Source: CAD feature listing. Evaluate the final solid. Frame: model axes, mm. A direction names the side the tool comes from. Round coordinates to 2 decimals unless told otherwise and drop trailing zeros. Order: outer loops, then holes, each group sorted by start corner. A loop starts at its lowest first (then second) coordinate and runs counter-clockwise, first axis right, second up.
Autodesk Inventor part; units mm, degrees
ref_plane "YZ Plane" through (0, 0, 0) normal (1, 0, 0) x (0, 1, 0)
ref_plane "XZ Plane" through (0, 0, 0) normal (0, 1, 0) x (-1, 0, 0)
ref_plane "XY Plane" through (0, 0, 0) normal (0, 0, 1) x (1, 0, 0)
ref_plane "Arbeitsebene1" through (-0.5, 0, -8) normal (0, -1, 0) x (1, 0, 0)
sketch "Skizze1" plane through (-0.5, 0, -8) normal (0, -1, 0) x (1, 0, 0)
  line L0 (-6.1, 20) -> (0.5, 20)
  line L1 (0.5, 20) -> (0.5, -4)
  line L2 (0.5, -4) -> (-6.1, -4)
  line L3 (-6.1, -4) -> (-6.1, 20)
  line L4 (0.5, 0) -> (32.9, 0)
  line L5 (0.5, 16) -> (34.9, 16)
  line L6 (0.5, 0) -> (34.9, 0)
  line L7 (34.9, 0) -> (34.9, 16)
  line L8 (34.9, 16) -> (0.5, 16)
  line L9 (0.5, 16) -> (0.5, 0)
  circle A0 centre (5.5, 8) radius 1.6
  circle A1 centre (5.5, 8) radius 1.6
  circle A2 centre (20.5, 8) radius 1.6
  circle A3 centre (20.5, 8) radius 1.6
  circle A4 centre (5.5, 8) radius 2.75
  circle A5 centre (20.5, 8) radius 2.75
  point P0 (0.5, 8)
  dimension "d0" = 5.5
  dimension "d1" = 5.5
extrude "Extrusion1" add sketch "Skizze1" along normal blind 10 contours L0 L1 L2 L3 | L5 L7 L6 L4 L1 | A4 | A5
ref_plane "Arbeitsebene2" through (-6.6, 0, -12) normal (-1, 0, 0) x (0, 0, 1)
sketch "Skizze2" plane through (-6.6, 0, -12) normal (-1, 0, 0) x (0, 0, 1)
  line L0 (0, -10) -> (4, -10)
  line L1 (0, -10) -> (24, -10)
  line L2 (24, -10) -> (24, -25)
  line L3 (24, -25) -> (0, -25)
  line L4 (0, -25) -> (0, -10)
  line L5 (0, 0) -> (0, -10)
  line L6 (0, 0) -> (4, 0)
  line L7 (0, -10) -> (2, -10)
  line L8 (2, -10) -> (2, 0)
  line L9 (2, 0) -> (0, 0)
  line L10 (0, 0) -> (0, -10)
  line L11 (4, 0) -> (4, -10)
  line L12 (4, -10) -> (20, -10)
  line L13 (20, -10) -> (20, -20)
  line L14 (20, -20) -> (4, -20)
  line L15 (4, -20) -> (4, -10)
  line L16 (4, -10) -> (5.5, -10)
  line L17 (5.5, -10) -> (5.5, -20)
  line L18 (5.5, -20) -> (4, -20)
  line L19 (4, -20) -> (4, -10)
  circle A0 centre (12, -25) radius 16.3478
  line L20 (12, -8.6522) -> (12, -5.6522)
  line L21 (12, -5.6522) -> (12, -3.6522)
  circle A1 centre (12, -25) radius 19.3478
  circle A2 centre (12, -25) radius 21.3478
  line L22 (4, -20) -> (20, -20)
  line L23 (20, -20) -> (20, 0)
  line L24 (20, 0) -> (4, 0)
  line L25 (4, 0) -> (4, -20)
  point P0 (12, 0)
  point P1 (18.5, -10)
  point P2 (20, -7.3836)
  point P3 (20, -5.2079)
  point P4 (4, -5.2079)
  point P5 (4, -7.3836)
  dimension "d4" = 15
  dimension "d5" = 16
  dimension "d6" = 10
  dimension "d7" = 1.5
  dimension "d14" = 3
  dimension "d15" = 2
extrude "Extrusion2" cut sketch "Skizze2" against normal up to surface (41 mm away) contours A0 L1
sketch "Skizze4" plane through (-0.5, -10, -8) normal (0, -1, 0) x (1, 0, 0)
  circle A0 centre (20.5, 8) radius 1.6
  circle A1 centre (20.5, 8) radius 2.8
  circle A2 centre (5.5, 8) radius 1.6
  circle A3 centre (5.5, 8) radius 2.8
  line L0 (7.1166, 10.8) -> (8.7332, 8)
  line L1 (8.7332, 8) -> (7.1166, 5.2)
  line L2 (7.1166, 5.2) -> (3.8834, 5.2)
  line L3 (3.8834, 5.2) -> (2.2668, 8)
  line L4 (2.2668, 8) -> (3.8834, 10.8)
  line L5 (3.8834, 10.8) -> (7.1166, 10.8)
  line L6 (22.1166, 10.8) -> (23.7332, 8)
  line L7 (23.7332, 8) -> (22.1166, 5.2)
  line L8 (22.1166, 5.2) -> (18.8834, 5.2)
  line L9 (18.8834, 5.2) -> (17.2668, 8)
  line L10 (17.2668, 8) -> (18.8834, 10.8)
  line L11 (18.8834, 10.8) -> (22.1166, 10.8)
  point P0 (0.5, 8)
  point P1 (5.5, 10.8)
  point P2 (20.5, 10.8)
  dimension "d29" = 5.6
  dimension "d30" = 5.6
extrude "Extrusion3" cut sketch "Skizze4" against normal blind 5 contours A0 | A1 | A1 L6 L7 | A1 L11 L6 | L7 L8 A1 | A1 L10 L11 | L8 L9 A1 | A1 L9 L10 | A2 | A3 | A3 L0 L1 | A3 L5 L0 | L1 L2 A3 | A3 L4 L5 | L2 L3 A3 | A3 L3 L4
extrude "Extrusion4" cut sketch "Skizze2" against normal blind 38 contours L11 A2 L21 A1 | A1 L21 A2 L23
extrude "Extrusion5" add sketch "Skizze2" against normal blind 32.5 contours L11 A2 L21 A1 | A1 L21 A2 L23
extrude "Extrusion6" cut sketch "Skizze2" against normal blind 22.05 contours L11 A2 L21 A1 | A1 L21 A2 L23
extrude "Extrusion7" add sketch "Skizze2" against normal blind 16.55 contours L11 A2 L21 A1 | A1 L21 A2 L23
extrude "Extrusion8" cut sketch "Skizze1" along normal blind 16.55 contours A0 | A2
extrude "Extrusion9" cut sketch "Skizze1" along normal blind 2 contours L0 L1 L2 L3 | L5 L7 L6 L4 L1 | A4 | A5
fillet "Rundung1" radius 0.5 9 edges at (-3.3, -10, 12) (0, -10, 10) (17.2, -10, 8) (34.4, -10, 7.25) (34.4, -8.6522, 0) (34.4, -10, -7.25) (17.2, -10, -8) (0, -10, -10) (-3.3, -10, -12)
sketch "Skizze6" plane through (34.4, -2, 8) normal (1, 0, 0) x (0, 0, -1)
  line L0 (-31.6615, 20.7831) -> (48.4189, 20.7831)
  line L1 (48.4189, 20.7831) -> (48.4189, -28.9012)
  line L2 (48.4189, -28.9012) -> (-31.6615, -28.9012)
  line L3 (-31.6615, -28.9012) -> (-31.6615, 20.7831)
  point P0 (8, 2)
extrude "Extrusion10" cut sketch "Skizze6" against normal blind 9
sketch "Skizze7" plane through (-6.6, -25, 0) normal (-1, 0, 0) x (0, 0, 1)
  line L0 (-50.9718, 43.6316) -> (27.5939, 43.6316)
  line L1 (27.5939, 43.6316) -> (27.5939, 3.9448)
  line L2 (27.5939, 3.9448) -> (-50.9718, 3.9448)
  line L3 (-50.9718, 3.9448) -> (-50.9718, 43.6316)
  point P0 (0, 25)
extrude "Extrusion11" cut sketch "Skizze7" against normal blind 6.6
properties part number "OBS-Displaymountadapter_schmal"
1. Section B-B on y = -3.25. Return loops of the section in (x, z).
2. Section C-C on z = 5. Return loops of the section in (x, y), plus the area to 3 significant figures.
3. Section A-A on x = 5. Return loops of the section in (y, z), plus the area to 3 significant figures.
4. Line query: line 1 along X through (y, z) = (-2.85, 0); line 2 along X through (y, z) = (-3.85, 0); line 3 along Z through (x, y) = (20, -3.85). Output: solid intervals per line, ascending.
5. Pull-direction query (Z, two-part tool) for faces 4 (the face through (0, -6, 0)), 5 (the face through (5, -7, 2.8)), 6 (the face through (13, -5, -8)); classes: released by +Z, released by -Z, zero draft, split by the parting line, or undercut.
6. Section D-D on y = -9.25. Return loops of the section in (x, z).
7. First-contact query: pin 1 (3 mm diameter, centred on x = 20, z = 0, fed in from -Y); pin 2 (5 mm diameter, centred on x = 5, z = 0, fed in from +Y). Flat tips, straight axial feed; report the tip coordinate or a pass-through.
8. Access query for faces 1 (the face through (13, -2, 0)), 2 (the face through (6.392, -5.695, 1.287)), 3 (the face through (9.95, -5, 0)). Directions: +Z, -Z, +X, -X, +Y, -Y. A direction counts if a zero-diameter tool reaches every point of the face in a straight line with its end or side. Return the directions, or none.
Result:
1. outline: (0, -8) - (25.4, -8) - (25.4, 8) - (0, 8) - close; hole circle Ø3.2 at (5, 0); hole circle Ø3.2 at (20, 0)
2. outline: (0, -9.44) - (25.4, -9.44) - (25.4, -2) - (0, -2) - close; hole (9.95, -6.31) - (15.45, -6.31) - (15.45, -4.25) - (9.95, -4.25) - close
2. area: 178 mm2
3. outline: (-10, -7.5) arc R0.5 ccw to (-9.5, -8) - (-2, -8) - (-2, -1.6) - (-5.72, -1.6) arc R19.35 cw to (-5.86, -2.8) - (-8.89, -2.8) arc R16.35 cw to (-10, -6.5) - close; (-10, 6.5) arc R16.35 cw to (-8.89, 2.8) - (-5.86, 2.8) arc R19.35 cw to (-5.72, 1.6) - (-2, 1.6) - (-2, 8) - (-9.5, 8) arc R0.5 ccw to (-10, 7.5) - close
3. area: 87.5 mm2
4. line 1: x = 0 to 3.4, 6.6 to 18.4, 21.6 to 25.4
4. line 2: x = 0 to 3.4, 6.6 to 9.95, 15.45 to 18.4, 21.6 to 25.4
4. line 3: z = -8 to -1.6, 1.6 to 8
5. face 4: zero draft
5. face 5: undercut
5. face 6: released by -Z
6. outline: (0, -8) - (25.4, -8) - (25.4, -4.38) - (0, -4.38) - close; (0, 4.38) - (25.4, 4.38) - (25.4, 8) - (0, 8) - close
7. pin 1: passes through
7. pin 2: stops at y = -2
8. face 1: +Z, -Z, +X, -X, +Y
8. face 2: -Y
8. face 3: none
